For this review, take the finished solid that the model builds, in its own axes (mm). Coordinates: 2 decimals unless noted, no trailing zeros. Write each loop counter-clockwise with the first axis right and the second up, starting at its lowest first coordinate (ties: lowest second). Pieces come first, ordered by that corner, then holes. Notation, with made-up numbers: (44, 35) - (98, 35) arc R30 ccw to (98, 69) - close; hole circle Ø7 at (12, 87). An arc over 180 degrees is marked (long way). Use one line per item in the form item = value. Start each with the question number.
1) For L1, parallel to Y at x = 0, z = 13.25; L2, parallel to Z at x = -1.9, y = -0.15; L3, parallel to Y at x = -2.3, z = -0.5, list the stretches that pass through material, from the lowest coordinate up. Write a range as from..to.
2) Mouldability with a two-part tool opening along X and no side actions: class faces 1 (the flat face through (0, 0, -1.15)), 2 (the flat face through (-1.2, -1.2, 0)), 3 (the cylindrical face through (-1.5, 0.07, 6.9)) as pulls with the +X half, pulls with the -X half, needs draft (parallel to the pull), parting line crosses it, or undercut.
3) We need section A-A (z = 9.75). Give the boundary of the cut face in (x, y).
4) Insertion check: P1, Ø1, axis at x = -1, z = 3, coming from the +Y side; P2, Ø0.6, axis at y = 1, z = -1.5, coming from the -X side; P3, Ø2, axis at y = 0, z = 6, coming from the -X side. Each pin has a flat end and moves straight along its axis. Give the tip position at first contact, or say it passes through.
```python
from build123d import *

# Parameters (mm, degrees)
SKETCH_1_R          = 1.5
EXTRUDE_1_DEPTH     = 14
SKETCH_2_R          = 2.85
EXTRUDE_2_DEPTH     = 1.65
FILLET_1_R          = 2
CUT_EXTRUDE_1_DEPTH = 0.5


with BuildPart() as part:
    # 草图1 → 凸台-拉伸1 (new body)
    with BuildSketch(Plane.XY):
        Circle(SKETCH_1_R)
    extrude(amount=EXTRUDE_1_DEPTH)

    # 草图2 → 凸台-拉伸2 (add)
    with BuildSketch(Plane(origin=(0, 0, 0), x_dir=(-1, 0, 0), z_dir=(0, 0, -1))):
        Circle(SKETCH_2_R)
    extrude(amount=EXTRUDE_2_DEPTH)

    # 圆角1
    # the kernel refuses this fillet: 2 mm, written as the material it takes off along each edge
    with BuildSketch(Plane(origin=(0, 0, -1.65), x_dir=(-1, 0, 0), z_dir=(0, -1, 0))) as fillet_1_piece_1:
        with BuildLine():
            CenterArc((0.880863133, -2), FILLET_1_R, 10.078658108, 79.921341892)
            Line((0.880863133, 0), (0.880863133, 0.04))
            Line((0.880863133, 0.04), (2.85, 0.04))
            Line((2.85, 0.04), (2.89, 0))
            ThreePointArc((2.89, 0), (2.89, -0.825), (2.889382737, -1.643))
            Line((2.889382737, -1.643), (2.85, -1.65))
        make_face()
    revolve(axis=Axis((0, 0, -1.65), (0, 0, -1)), mode=Mode.SUBTRACT)

    # 草图3 → 切除-拉伸1 (cut)
    with BuildSketch(Plane(origin=(0, 0, -1.65), x_dir=(-1, 0, 0), z_dir=(0, 0, -1))):
        Polygon((2.85, 0.25), (2.85, -0.25), (0.25, -0.25), (0.25, -2.85), (-0.25, -2.85), (-0.25, -0.25), (-2.85, -0.25), (-2.85, 0.25), (-0.25, 0.25), (-0.25, 2.85), (0.25, 2.85), (0.25, 0.25), align=None)
    extrude(amount=-CUT_EXTRUDE_1_DEPTH, mode=Mode.SUBTRACT)


solid = part.part
```
Determined:
q1.L1 = -1.5..1.5
q1.L2 = -1.15..0
q1.L3 = -1.4..1.4
q2.face_1 = undercut
q2.face_2 = needs draft
q2.face_3 = parting line crosses it
q3.outline = circle Ø3 at (0, 0)
q4.P1 = 1.41
q4.P2 = -1.92
q4.P3 = -1.5
